Input: part model. Units: mm. Frame: model coordinates. Face numbers are marked on the shaded views. Give positions to 0.01 mm unless a question says otherwise; leave off trailing zeros. Order: outer loops, then holes, each group sorted by start corner. A loop starts at its lowest first (then second) coordinate and runs counter-clockwise, first axis right, second up. Notation, with made-up numbers: (-16, 32) -> (0, 32) arc R15 cw to (0, 38) -> close; hole circle Ø9 at (3.25, 11.5). An arc over 180 degrees is marked (long way). Use a Markdown table: item, result. Add a question column.
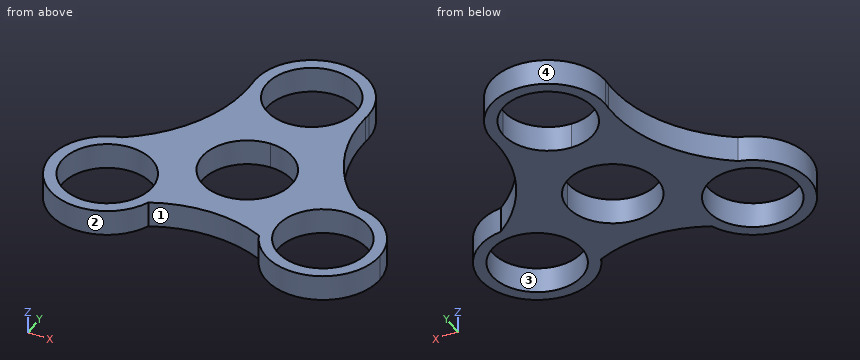
from build123d import *

# Parameters (mm, degrees)
F0_R     = 11.049
F1_DEPTH = 6.35


with BuildPart() as f1:
    # F0 (on Top) → F1 (new body)
    with BuildSketch(Plane.XY):
        with BuildLine():
            ThreePointArc((0, 11.049), (-7.812823, -7.812823), (11.049, 0))
            ThreePointArc((11.049, 0), (7.812823, 7.812823), (0, 11.049))
        make_face()
        with BuildLine():
            ThreePointArc((13.893866, 29.023504), (9.349162, 20.099534), (0, 16.51))
            ThreePointArc((0, 16.51), (-9.302947, 20.058096), (-13.880375, 28.900097))
            ThreePointArc((-13.880375, 28.900097), (-17.809173, 11.527031), (-29.759522, -1.680845))
            ThreePointArc((-29.759522, -1.680845), (-17.788933, -4.236751), (-12.426454, -15.24))
            ThreePointArc((-12.426454, -15.24), (-12.702084, -18.001363), (-13.518097, -20.653762))
            ThreePointArc((-13.518097, -20.653762), (-0.046654, -17.568603), (13.457498, -20.507288))
            ThreePointArc((13.457498, -20.507288), (15.296029, -6.758169), (28.078999, -1.371693))
            ThreePointArc((28.078999, -1.371693), (17.354133, 12.130747), (13.893866, 29.023504))
        make_face()
        with BuildLine():
            ThreePointArc((0, 11.049), (7.812823, 7.812823), (11.049, 0))
            ThreePointArc((11.049, 0), (-7.812823, -7.812823), (0, 11.049))
        make_face(mode=Mode.SUBTRACT)
        with BuildLine():
            ThreePointArc((11.049, 30.48), (-7.812823, 38.292823), (0, 19.431))
            ThreePointArc((0, 19.431), (7.812823, 22.667177), (11.049, 30.48))
        make_face()
        with BuildLine():
            ThreePointArc((-13.880375, 28.900097), (-9.302947, 20.058096), (0, 16.51))
            ThreePointArc((0, 16.51), (9.349162, 20.099534), (13.893866, 29.023504))
            ThreePointArc((13.893866, 29.023504), (13.924773, 29.752126), (13.97, 30.48))
            ThreePointArc((13.97, 30.48), (0, 44.45), (-13.97, 30.48))
            ThreePointArc((-13.97, 30.48), (-13.916283, 29.690554), (-13.880375, 28.900097))
        make_face()
        with BuildLine():
            ThreePointArc((11.049, 30.48), (7.812823, 22.667177), (0, 19.431))
            ThreePointArc((0, 19.431), (-7.812823, 38.292823), (11.049, 30.48))
        make_face(mode=Mode.SUBTRACT)
        with BuildLine():
            ThreePointArc((-13.97, 30.48), (-13.947576, 29.688778), (-13.880375, 28.900097))
            ThreePointArc((-13.880375, 28.900097), (-13.916283, 29.690554), (-13.97, 30.48))
        make_face()
        with BuildLine():
            ThreePointArc((13.97, 30.48), (13.924773, 29.752126), (13.893866, 29.023504))
            ThreePointArc((13.893866, 29.023504), (13.950954, 29.750758), (13.97, 30.48))
        make_face()
        with BuildLine():
            ThreePointArc((-12.426454, -15.24), (-17.788933, -4.236751), (-29.759522, -1.680845))
            ThreePointArc((-29.759522, -1.680845), (-37.009092, -24.324758), (-13.518097, -20.653762))
            ThreePointArc((-13.518097, -20.653762), (-12.702084, -18.001363), (-12.426454, -15.24))
        make_face()
        with Locations((-26.396454, -15.24)):
            Circle(F0_R, mode=Mode.SUBTRACT)
        with BuildLine():
            ThreePointArc((40.366454, -15.24), (36.852698, -5.975667), (28.078999, -1.371693))
            ThreePointArc((28.078999, -1.371693), (15.296029, -6.758169), (13.457498, -20.507288))
            ThreePointArc((13.457498, -20.507288), (29.080079, -28.949816), (40.366454, -15.24))
        make_face()
        with Locations((26.396454, -15.24)):
            Circle(F0_R, mode=Mode.SUBTRACT)
    extrude(amount=F1_DEPTH)


solid = f1.part
Q1. Ray query, line 1 (Y direction, x = 10, z = 3.25); line 2 (X direction, y = -24, z = 3); line 3 (Y direction, x = -3, z = 0.5). Return the intervals inside material, ascending.
Q2. First-contact query: pin 1 (1 mm diameter, centred on y = -15, z = 3, fed in from -X); pin 2 (1.5 mm diameter, centred on y = 34, z = 5, fed in from +X); pin 3 (3 mm diameter, centred on y = 30.5, z = 4, fed in from -X); pin 4 (2 mm diameter, centred on y = 22, z = 5.5, fed in from -X). Flat tips, straight axial feed; report the tip coordinate or a pass-through.
Q3. Section query A-A (x = -25.5). Return loops of the section in (y, z), plus the area to 3 significant figures.
Q4. Draft query along Y for the marked faces 1, 2, 3 and 4. Return one class per face: +Y half, -Y half, draft (parallel to the pull), parting line (faces both ways), or undercut.
Q5. Section query B-B (y = 36). Return loops of the section in (x, z), plus the area to 3 significant figures.
Q6. Section query C-C (z = 5). Return loops of the section in (x, y), plus the area to 3 significant figures.
Q7. Section query D-D (y = -12). Return loops of the section in (x, z).
Solution:
| question | item | result |
|---|---|---|
| 1 | line 1 | y = -19.14 to -4.7, 4.7 to 25.78, 35.18 to 40.24 |
| 1 | line 2 | x = -37.28 to -33.13, -19.66 to -15.51, 15.51 to 19.66, 33.13 to 37.28 |
| 1 | line 3 | y = -17.72 to -10.63, 10.63 to 19.85, 41.11 to 44.12 |
| 2 | pin 1 | stops at x = -40.37 |
| 2 | pin 2 | stops at x = 13.69 |
| 2 | pin 3 | stops at x = -13.97 |
| 2 | pin 4 | stops at x = -14.51 |
| 3 | outline | (-29.18, 0) -> (-26.25, 0) -> (-26.25, 6.35) -> (-29.18, 6.35) -> close; (-4.23, 0) -> (1.59, 0) -> (1.59, 6.35) -> (-4.23, 6.35) -> close |
| 3 | area | 55.6 mm² |
| 4 | face 1 | -Y half |
| 4 | face 2 | parting line |
| 4 | face 3 | undercut |
| 4 | face 4 | +Y half |
| 5 | outline | (-12.83, 0) -> (-9.57, 0) -> (-9.57, 6.35) -> (-12.83, 6.35) -> close; (9.57, 0) -> (12.83, 0) -> (12.83, 6.35) -> (9.57, 6.35) -> close |
| 5 | area | 41.4 mm² |
| 6 | outline | (-29.76, -1.68) arc R13.97 ccw (long way) to (-13.52, -20.65) arc R31.71 cw to (13.46, -20.51) arc R13.97 ccw (long way) to (28.08, -1.37) arc R37.09 cw to (13.89, 29.02) arc R13.97 ccw to (13.97, 30.48) arc R13.97 ccw to (-13.97, 30.48) arc R13.97 ccw to (-13.88, 28.9) arc R35.1 cw to start; hole circle Ø22.1 at (-26.4, -15.24); hole circle Ø22.1 at (0, 0); hole circle Ø22.1 at (0, 30.48); hole circle Ø22.1 at (26.4, -15.24) |
| 6 | area | 1,650 mm² |
| 7 | outline | (-39.99, 0) -> (-36.96, 0) -> (-36.96, 6.35) -> (-39.99, 6.35) -> close; (-15.83, 0) -> (15.83, 0) -> (15.83, 6.35) -> (-15.83, 6.35) -> close; (36.96, 0) -> (39.99, 0) -> (39.99, 6.35) -> (36.96, 6.35) -> close |
